Read the model definition and answer for the solid it produces. Units are mm, in the model's axes. A direction names the side the tool comes from. Give positions to 0.01 mm unless a question says otherwise; leave off trailing zeros. Order: outer loops, then holes, each group sorted by start corner. A loop starts at its lowest first (then second) coordinate and runs counter-clockwise, first axis right, second up. Notation, with made-up numbers: (74.5, 19.5) - (130.5, 19.5) arc R34 cw to (130.5, 58.5) - close; hole circle Ø4 at (-13, -0.5). An arc over 180 degrees is marked (long way). Write each question's results on one line, items separated by ' | '.
from build123d import *

# Parameters (mm, degrees)
BOSS_EXTRUDE1_DEPTH = 304.8
SKETCH4_R           = 4.826
CUT_EXTRUDE1_DEPTH  = 309.273534432


with BuildPart() as part:
    # Sketch1 → Boss-Extrude1 (new body)
    with BuildSketch(Plane.XY):
        with BuildLine():
            Line((-36.22675, 20.6375), (-3.46075, 20.6375))
            ThreePointArc((-3.46075, 20.6375), (-1.013630207, 19.623869793), (0, 17.17675))
            Line((0, 17.17675), (0, -17.17675))
            ThreePointArc((0, -17.17675), (-1.013630207, -19.623869793), (-3.46075, -20.6375))
            Line((-3.46075, -20.6375), (-36.22675, -20.6375))
            ThreePointArc((-36.22675, -20.6375), (-39.796401808, -19.158901808), (-41.275, -15.58925))
            Line((-41.275, -15.58925), (-41.275, -14.57325))
            ThreePointArc((-41.275, -14.57325), (-40.261369793, -12.126130207), (-37.81425, -11.1125))
            Line((-37.81425, -11.1125), (-35.5346, -11.1125))
            ThreePointArc((-35.5346, -11.1125), (-34.1376, -12.5095), (-35.5346, -13.9065))
            Line((-35.5346, -13.9065), (-37.81425, -13.9065))
            ThreePointArc((-37.81425, -13.9065), (-38.285713446, -14.101786554), (-38.481, -14.57325))
            Line((-38.481, -14.57325), (-38.481, -15.58925))
            ThreePointArc((-38.481, -15.58925), (-37.820745461, -17.183245461), (-36.22675, -17.8435))
            Line((-36.22675, -17.8435), (-3.46075, -17.8435))
            ThreePointArc((-3.46075, -17.8435), (-2.989286554, -17.648213446), (-2.794, -17.17675))
            Line((-2.794, -17.17675), (-2.794, 17.17675))
            ThreePointArc((-2.794, 17.17675), (-2.989286554, 17.648213446), (-3.46075, 17.8435))
            Line((-3.46075, 17.8435), (-36.22675, 17.8435))
            ThreePointArc((-36.22675, 17.8435), (-37.820745461, 17.183245461), (-38.481, 15.58925))
            Line((-38.481, 15.58925), (-38.481, 14.57325))
            ThreePointArc((-38.481, 14.57325), (-38.285713446, 14.101786554), (-37.81425, 13.9065))
            Line((-37.81425, 13.9065), (-35.5346, 13.9065))
            ThreePointArc((-35.5346, 13.9065), (-34.1376, 12.5095), (-35.5346, 11.1125))
            Line((-35.5346, 11.1125), (-37.81425, 11.1125))
            ThreePointArc((-37.81425, 11.1125), (-40.261369793, 12.126130207), (-41.275, 14.57325))
            Line((-41.275, 14.57325), (-41.275, 15.58925))
            ThreePointArc((-41.275, 15.58925), (-39.796401808, 19.158901808), (-36.22675, 20.6375))
        make_face()
    extrude(amount=-BOSS_EXTRUDE1_DEPTH)

    # Sketch4 → Cut-Extrude1 (cut, through all)
    with BuildSketch(Plane(origin=(0, 0, 0), x_dir=(0, 0, -1), z_dir=(1, 0, 0))):
        with Locations(Location((152.4, 0, 0), (0, 0, 90))):
            Circle(SKETCH4_R)
    extrude(amount=-CUT_EXTRUDE1_DEPTH, mode=Mode.SUBTRACT)


solid = part.part
(1) For faces 1 (the face through (-2.794, -8, -150)), 2 (the face through (-20, -20.638, -150)), determine the directions among +Z, -Z, +X, -X, +Y, -Y from which every point of the face is accessible in a straight line to the end or side of a thin tool.
Conclusion:
face 1: +Z, -Z | face 2: +Z, -Z, +X, -X, -Y
(2) Section D-D (z = -253) is taken. Give the vertices of the cut face in (x, y) (1 decimal), plus the area to 3 significant figures.
Conclusion:
outline: (-41.3, -15.6) arc R5 ccw to (-36.2, -20.6) - (-3.5, -20.6) arc R3.5 ccw to (0, -17.2) - (0, 17.2) arc R3.5 ccw to (-3.5, 20.6) - (-36.2, 20.6) arc R5 ccw to (-41.3, 15.6) - (-41.3, 14.6) arc R3.5 ccw to (-37.8, 11.1) - (-35.5, 11.1) arc R1.4 ccw to (-35.5, 13.9) - (-37.8, 13.9) arc R0.7 cw to (-38.5, 14.6) - (-38.5, 15.6) arc R2.3 cw to (-36.2, 17.8) - (-3.5, 17.8) arc R0.7 cw to (-2.8, 17.2) - (-2.8, -17.2) arc R0.7 cw to (-3.5, -17.8) - (-36.2, -17.8) arc R2.3 cw to (-38.5, -15.6) - (-38.5, -14.6) arc R0.7 cw to (-37.8, -13.9) - (-35.5, -13.9) arc R1.4 ccw to (-35.5, -11.1) - (-37.8, -11.1) arc R3.5 ccw to (-41.3, -14.6) - close | area: 372 mm^2
(3) Each of these flat-tipped pins is pushed along its axis until it touches: pin 1 (1.8 mm diameter, centred on x = -37, z = -161.5, fed in from -Y); pin 2 (2 mm diameter, centred on x = -32, y = 13.5, fed in from +Z); pin 3 (6 mm diameter, centred on y = -3.5, z = -86.5, fed in from -X). Where does it stop, or does it pass through?
Conclusion:
pin 1: y = -20.64 | pin 2: through | pin 3: x = -2.79
(4) Section C-C (y = 0) is taken. Give the vertices of the cut face in (x, z), plus the area to 3 significant figures.
Conclusion:
outline: (-2.79, -304.8) - (0, -304.8) - (0, -157.23) - (-2.79, -157.23) - close; (-2.79, -147.57) - (0, -147.57) - (0, 0) - (-2.79, 0) - close | area: 825 mm^2
(5) The mould has two halves that part along X. Classify faces 3 (the face through (0, 8, -150)), 4 (the face through (-20, -17.844, -150)), 5 (the face through (-39.835, 19.119, -150.266)), 6 (the face through (-2, 0, -304.8)): pulls with the +X half, pulls with the -X half, needs draft (parallel to the pull), parting line crosses it, or undercut.
Conclusion:
face 3: pulls with the +X half | face 4: undercut | face 5: pulls with the -X half | face 6: needs draft
(6) Consider probe 1 along Y at (x, z) = (-34, -26.5); probe 2 along X at (y, z) = (-14.5, -208); probe 3 along Z at (x, y) = (-1.25, 0). Determine where each line is inside the solid, lowest interval first. Write a range as [from, to].
Conclusion:
probe 1: [-20.64, -17.84], [17.84, 20.64] | probe 2: [-41.27, -38.48], [-2.79, 0] | probe 3: [-304.8, -157.23], [-147.57, 0]
(7) Section B-B (x = -14.5) is taken. Give the vertices of the cut face in (y, z), plus the area to 3 significant figures.
Conclusion:
outline: (-20.64, -304.8) - (-17.84, -304.8) - (-17.84, 0) - (-20.64, 0) - close; (17.84, -304.8) - (20.64, -304.8) - (20.64, 0) - (17.84, 0) - close | area: 1,700 mm^2
